Check sheet for the modelled part. Datum: model origin and axes. Units: mm. Face numbers are marked on the shaded views. A direction names the side the tool comes from. Coordinates: 2 decimals unless noted, no trailing zeros. Order: outer loops, then holes, each group sorted by start corner. A loop starts at its lowest first (then second) coordinate and runs counter-clockwise, first axis right, second up.
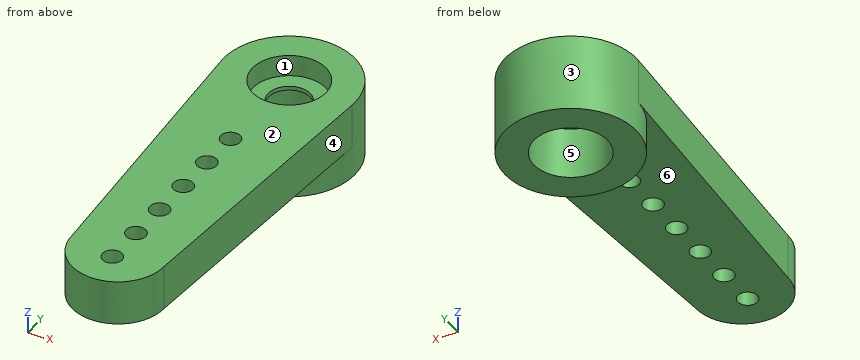
from build123d import *

# Parameters (mm, degrees)
SKETCH1_R           = 3.5687
SKETCH1_R_2         = 2
BOSS_EXTRUDE1_DEPTH = 4.191
SKETCH5_R           = 2
SKETCH5_R_2         = 1.143
BOSS_EXTRUDE2_DEPTH = 0.2226
BOSS_EXTRUDE3_START = -2.441
SKETCH6_R           = 0.5334
BOSS_EXTRUDE3_DEPTH = 2.441


with BuildPart() as part:
    # Sketch1 → Boss-Extrude1 (new body)
    with BuildSketch(Plane.XY.offset(-7.032965862)):
        Circle(SKETCH1_R)
        Circle(SKETCH1_R_2, mode=Mode.SUBTRACT)
    extrude(amount=BOSS_EXTRUDE1_DEPTH)

    # Sketch5 → Boss-Extrude2 (add)
    with BuildSketch(Plane.XY.offset(-4.232965862)):
        Circle(SKETCH5_R)
        Circle(SKETCH5_R_2, mode=Mode.SUBTRACT)
    extrude(amount=BOSS_EXTRUDE2_DEPTH)

    # Sketch6 → Boss-Extrude3 (add)
    with BuildSketch(Plane.XY.offset(-2.841965862).offset(BOSS_EXTRUDE3_START)):
        with BuildLine():
            Line((2.5, -15.9313), (3.56, -0.249037527))
            ThreePointArc((3.56, -0.249037527), (0, -3.5687), (-3.56, -0.249037527))
            Line((-3.56, -0.249037527), (-2.5, -15.9313))
            ThreePointArc((-2.5, -15.9313), (0, -18.4313), (2.5, -15.9313))
        make_face()
        with Locations((0, -14.2647)):
            Circle(SKETCH6_R, mode=Mode.SUBTRACT)
        with Locations((0, -16.4647)):
            Circle(SKETCH6_R, mode=Mode.SUBTRACT)
        with Locations((0, -12.0647)):
            Circle(SKETCH6_R, mode=Mode.SUBTRACT)
        with Locations((0, -9.8647)):
            Circle(SKETCH6_R, mode=Mode.SUBTRACT)
        with Locations((0, -7.6647)):
            Circle(SKETCH6_R, mode=Mode.SUBTRACT)
        with Locations((0, -5.4647)):
            Circle(SKETCH6_R, mode=Mode.SUBTRACT)
    extrude(amount=BOSS_EXTRUDE3_DEPTH)


solid = part.part
(1) Release check for a two-part mould opening along Y. For the marked faces 4, 5 and 6 record: +Y half, -Y half, draft (parallel to the pull), parting line (faces both ways), or undercut.
Filled in:
face 4: -Y half
face 5: undercut
face 6: draft
(2) Go/stop test with flat-tipped pins: P1, Ø2, axis at x = -0.5, y = 1, coming from the -Z side; P2, Ø3, axis at x = 0, y = 0, coming from the +Z side; P3, Ø2, axis at x = -0.5, y = -5.5, coming from the -Z side; P4, Ø2.5, axis at x = 0, y = 0, coming from the -Z side. Record where each tip stops, or that it passes through.
Filled in:
P1: stops at z = -7.03
P2: stops at z = -4.01
P3: stops at z = -5.28
P4: stops at z = -4.23
(3) Cross-section at D-D (x = 1.5). Enter the section's corners in (y, z).
Filled in:
outline: (-17.93, -5.28) - (-3.24, -5.28) - (-3.24, -7.03) - (-1.32, -7.03) - (-1.32, -4.23) - (1.32, -4.23) - (1.32, -7.03) - (3.24, -7.03) - (3.24, -2.84) - (1.32, -2.84) - (1.32, -4.01) - (-1.32, -4.01) - (-1.32, -2.84) - (-17.93, -2.84) - close
(4) Cross-section at B-B (x = 0). Count the separate pieces of the cut face and the enclosed holes in it, and give its area (3 significant figures).
Filled in:
separate pieces: 8
enclosed holes: 0
area: 34.2 mm2
(5) Thickness scan on probe 1 along Z at (x, y) = (-1.5, -4.75); probe 2 along Z at (x, y) = (1.5, 0.25); probe 3 along Y at (x, z) = (-0.25, -5.8). Record the ranges inside material, lowest first.
Filled in:
probe 1: z = -5.28 to -2.84
probe 2: z = -4.23 to -4.01
probe 3: y = -3.56 to -1.98, 1.98 to 3.56
(6) Tool access check on the marked faces 1, 2 and 3. Record the directions out of +Z, -Z, +X, -X, +Y, -Y that give a thin tool (end or side, any length) a straight path to the whole face; none if there is none.
Filled in:
face 1: +Z
face 2: +Z, +X, -X, +Y, -Y
face 3: -Z
(7) Cross-section at C-C (z = -6.15). Enter the section's corners in (x, y).
Filled in:
outline: circle Ø7.14 at (0, 0); hole circle Ø4 at (0, 0)
(8) Cross-section at A-A (y = 0). Enter the section's corners in (x, z), and give its area (3 significant figures).
Filled in:
outline: (-3.57, -7.03) - (-2, -7.03) - (-2, -4.23) - (-1.14, -4.23) - (-1.14, -4.01) - (-2, -4.01) - (-2, -2.84) - (-3.57, -2.84) - close; (1.14, -4.23) - (2, -4.23) - (2, -7.03) - (3.57, -7.03) - (3.57, -2.84) - (2, -2.84) - (2, -4.01) - (1.14, -4.01) - close
area: 13.5 mm2
